Work out the finished part from the listing and answer in its coordinate system (mm). Face numbers are marked on the shaded views. A direction names the side the tool comes from. Give positions to 0.01 mm unless a question says otherwise; leave off trailing zeros. Write each loop counter-clockwise with the first axis right and the second up, starting at its lowest first coordinate (ties: lowest second). Pieces come first, ordered by that corner, then holes. Notation, with made-up numbers: (74, -33.75) - (100, -33.75) arc R23 cw to (100, -5.75) - close; hole circle Ø3 at (31.25, 70.25). An arc over 180 degrees is marked (long way). Write each question's results on one line, items separated by ' | '. Start each with the question number.
Autodesk Inventor part; units mm, degrees
ref_plane "Work Plane1" through (3.5, 0, 0) normal (0, 0, 1) x (1, 0, 0)
ref_plane "YZ Plane" through (0, 0, 0) normal (1, 0, 0) x (0, 1, 0)
ref_plane "XZ Plane" through (0, 0, 0) normal (0, 1, 0) x (-1, 0, 0)
sketch "Sketch1" plane through (0, 0, 0) normal (0, 0, 1) x (1, 0, 0)
  line L0 (0, 5) -> (0, 2.0092)
  line L1 (1.6, 2.5) -> (10, 2.5)
  line L2 (10, 2.5) -> (10, 0)
  line L3 (10, 0) -> (-0.86, 0)
  line L4 (0, -1) -> (0, 6)
  line L5 (-3.032, 0) -> (12.172, 0)
  line L6 (-0.86, 0) -> (-0.86, 5)
  line L7 (-0.86, 5) -> (0, 5)
  line L8 (1.6, 2.5) -> (1.1092, 2.0092)
  line L9 (1.1092, 2.0092) -> (0, 2.0092)
  dimension "d0" = 10
  dimension "d1" = 8.4
  dimension "d2" = 5
  dimension "d8" = 0.86
  dimension "d9" = 10
  dimension "d15" = 4.0185
  dimension "d16" = 0.4908
revolve "Body" add sketch "Sketch1" angle 360 about axis through (10, 0, 0) along (-1, 0, 0)
sketch "Sketch2" plane through (0, 0, 0) normal (1, 0, 0) x (0, 0, -1)
  circle A0 centre (0, 0) radius 5
  line L0 (0, 4.0415) -> (3.5, 2.0207)
  line L1 (3.5, 2.0207) -> (3.5, -2.0207)
  line L2 (3.5, -2.0207) -> (0, -4.0415)
  line L3 (0, -4.0415) -> (-3.5, -2.0207)
  line L4 (-3.5, -2.0207) -> (-3.5, 2.0207)
  line L5 (-3.5, 2.0207) -> (0, 4.0415)
  circle A1 centre (0, 0) radius 5
  dimension "d10" = 7
extrude "Head" add sketch "Sketch2" against normal blind 4.51 contours L0 L1 L2 L3 L4 L5
sketch "Sketch3" plane through (0, 0, 0) normal (0, 0, 1) x (1, 0, 0)
  line L0 (-4.51, 3.15) -> (-4.51, 4.0415)
  line L1 (-4.51, 4.0415) -> (-3.9953, 4.0415)
  line L2 (-3.9953, 4.0415) -> (-4.51, 3.15)
  line L3 (-2.0945, 4.0415) -> (-4.51, 4.0415)
  line L4 (-4.51, 4.0415) -> (-4.51, 1.7321)
  line L5 (-0.86, 4.0415) -> (-4.51, 4.0415)
  line L6 (-4.51, 4.0415) -> (-4.51, 2.0207)
  line L7 (-5.24, 0) -> (-0.13, 0)
  dimension "d5" = 30
  dimension "d18" = 6.3
revolve "Chamfer1" cut sketch "Sketch3" angle 360 about axis through (-10, 0, 0) along (1, 0, 0)
thread "Thread"
chamfer "Chamfer2" distance 0.4908 distance2 0.4908 1 edges at (10, -2.5, 0) measured on face at (10, -0.7379, 0.3873)
ref_plane "Work Plane1" through (3.5, 0, 0) normal (0, 0, 1) x (1, 0, 0)
equation "\"d10\" = SW"
equation "\"d3\" = KOH"
equation "\"d13\" = GEL"
equation "\"d6\" = -0.5 * SPD + 0.5 * GD"
equation "\"d7\" = -0.5 * SPD + 0.5 * GD"
equation "\"d0\" = NLG"
equation "\"d1\" = GEL"
equation "\"d2\" = GD"
equation "\"d8\" = PHH"
equation "\"d9\" = LADI"
equation "\"d15\" = BDM"
equation "\"d16\" = GAL"
equation "\"d5\" = ANG1"
equation "\"d18\" = SW0"
equation "\"NLG\" = 10"
equation "\"GD\" = NND"
equation "\"BDM\" = NND - 1.2269 * PTC"
equation "\"KOH\" = 4.51"
equation "\"GEL\" = 8.4"
equation "\"LADI\" = 10"
equation "\"SW\" = 7"
equation "\"PHH\" = 0.86"
equation "\"SW0\" = 6.3"
equation "\"SPD\" = NND - 1.2269 * PTC"
equation "\"ANG1\" = 30deg"
equation "\"GAL\" = 0.61345 * PTC"
equation "\"GUL\" = 0.61345 * PTC"
equation "\"WFT\" = PHH"
equation "\"PTC\" = 0.8"
equation "\"THREADDIA\" = 5"
equation "\"E0\" = 1.155 * SW"
equation "\"TOA\" = 30deg"
equation "\"NND\" = 5"
equation "\"GD1\" = THREADDIA - 1.2269 * PTC"
equation "\"SDH\" = 5.7"
equation "\"KOH1\" = 3.65"
equation "\"SD2\" = NND"
equation "\"SD\" = 0"
equation "\"RR\" = 0.2"
properties part number "AS 1427 - M5 x 10" material "Steel, Mild"
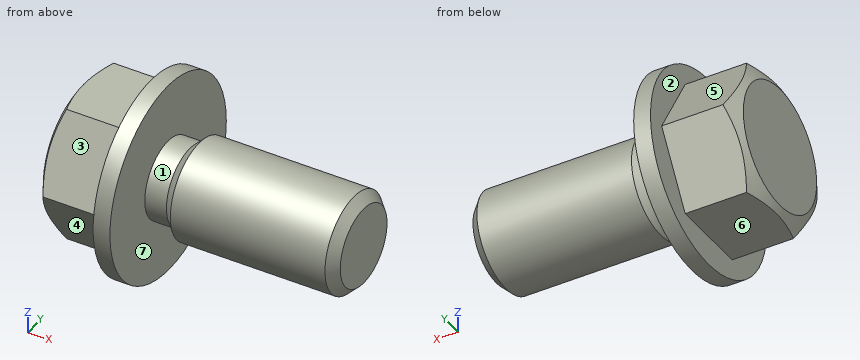
Q1. A cutting plane is placed at A-A, the plane y = 0. Write down the section's boundary in (x, z), and give its area (3 significant figures).
Q2. The mould has two halves that part along X. Classify the marked faces 1, 2 and 3: pulls with the +X half, pulls with the -X half, needs draft (parallel to the pull), parting line crosses it, or undercut.
Q3. A cutting plane is placed at C-C, the plane x = 0.25. Write down the section's boundary in (y, z).
Q4. Given pin 1 (2 mm diameter, centred on x = -3, y = -1.5, fed in from +Z); pin 2 (4 mm diameter, centred on x = -1, z = 3.5, fed in from -Y); pin 3 (6 mm diameter, centred on x = 1.5, y = -3, fed in from -Z), each flat-ended and moving along its own axis, determine where each tip first touches the part or whether it passes through.
Q5. A cutting plane is placed at D-D, the plane x = 8.5. Write down the section's boundary in (y, z).
Q6. A tool of negligible diameter and unlimited length cuts with its end or side. For the marked faces 4, 5, 6 and 7, from which of +Z, -Z, +X, -X, +Y, -Y can it reach the whole face along a straight path? Write none if from no direction.
Q7. Consider L1, parallel to X at y = -1.5, z = 2.75; L2, parallel to X at y = -2.75, z = 3.75; L3, parallel to Z at x = -1.75, y = 2. Determine where each line is inside the solid, lowest interval first.
Q8. A cutting plane is placed at B-B, the plane z = -4. Write down the section's boundary in (x, y).
Result:
1) outline: (-4.51, -3.15) - (-4.31, -3.5) - (-0.86, -3.5) - (-0.86, -5) - (0, -5) - (0, -2.01) - (1.11, -2.01) - (1.6, -2.5) - (9.51, -2.5) - (10, -2.01) - (10, 2.01) - (9.51, 2.5) - (1.6, 2.5) - (1.11, 2.01) - (0, 2.01) - (0, 5) - (-0.86, 5) - (-0.86, 3.5) - (-4.31, 3.5) - (-4.51, 3.15) - close | area: 82.5 mm2
2) face 1: undercut | face 2: pulls with the -X half | face 3: needs draft
3) outline: circle Ø4.02 at (0, 0)
4) pin 1: stops at z = 3.5 | pin 2: stops at y = -4.77 | pin 3: stops at z = -4.98
5) outline: circle Ø5 at (0, 0)
6) face 4: -Z, -X, -Y | face 5: +Z, -X, +Y | face 6: -Z, -X, +Y, -Y | face 7: none
7) L1: x = -4.51 to 0 | L2: x = -0.86 to 0 | L3: z = -3.5 to 3.5
8) outline: (-0.86, -3) - (0, -3) - (0, 3) - (-0.86, 3) - close
